Autodesk Inventor part; units mm, degrees
ref_plane "YZ Plane" through (0, 0, 0) normal (1, 0, 0) x (0, 1, 0)
ref_plane "XZ Plane" through (0, 0, 0) normal (0, 1, 0) x (-1, 0, 0)
ref_plane "XY Plane" through (0, 0, 0) normal (0, 0, 1) x (1, 0, 0)
sketch "Sketch1" plane through (0, 0, 0) normal (0, 0, 1) x (1, 0, 0)
  line L0 (-7, 0) -> (7, 0) construction
  line L1 (0, -2.8) -> (0, 2.8) construction
  line L2 (5, -2) -> (-5, -2)
  line L3 (-5, -2) -> (-5, 2)
  line L4 (-5, 2) -> (5, 2)
  line L5 (5, 2) -> (5, -2)
  line L6 (5, -2) -> (-5, 2) construction
  line L7 (-5, -2) -> (5, 2) construction
  point P0 (0, 0)
  dimension "d8" = 4
  dimension "d9" = 10
extrude "Extrusion1" add sketch "Sketch1" along normal blind 5
sketch "Sketch2" plane through (-5, 2, 0) normal (0, 1, 0) x (1, 0, 0)
  line L0 (10, 0) -> (10, -5)
  line L1 (10, 0) -> (0, 0)
  point P0 (5, 0)
  point P1 (7.5, -2.5)
  point P2 (10, -2.5)
  dimension "d12" = 2.5
hole "Hole1" at (2.5, 2, 2.5) direction (0, -1, 0) diameter 2.5 depth 10 tip angle 118 counterbore diameter 4 counterbore depth 2
sketch "Sketch3" plane through (-5, -2, 0) normal (0, -1, 0) x (1, 0, 0)
  circle A0 centre (7.5, 2.5) radius 1.25
  point P0 (5, 0)
  point P1 (2.5, 2.5)
  dimension "d21" = 5
hole "Hole2" at (-2.5, -2, 2.5) direction (0, 1, 0) diameter 2.5 depth 10 tip angle 118 counterbore diameter 4 counterbore depth 2
sketch "Sketch4" plane through (-5, 2, 0) normal (0, 1, 0) x (1, 0, 0)
  line L0 (0, 0) -> (0, -5)
  arc A0 (-12.5, 3.2297) -> (0, -2.5) centre (0, 14) ccw construction
  arc A1 (-14.3939, 1.5978) -> (0, -5) centre (0, 14) ccw
  arc A2 (-10.6061, 4.8615) -> (0, 0) centre (0, 14) ccw
  arc A3 (-10.6061, 4.8615) -> (-14.3939, 1.5978) centre (-12.5, 3.2297) ccw construction
  line L1 (10, 0) -> (0, 0)
  line L2 (10, -5) -> (0, -5)
  arc A4 (-12.5, 3.2297) -> (-27.5, 9.5) centre (-26.2704, -8.6352) ccw construction
  arc A5 (-10.6061, 4.8615) -> (-27.6691, 11.9943) centre (-26.2704, -8.6352) ccw
  arc A6 (-14.3939, 1.5978) -> (-27.3309, 7.0057) centre (-26.2704, -8.6352) ccw
  arc A7 (-14.3939, 1.5978) -> (-10.6061, 4.8615) centre (-12.5, 3.2297) ccw construction
  arc A8 (-27.6691, 11.9943) -> (-27.3309, 7.0057) centre (-27.5, 9.5) ccw
  circle A9 centre (2.5, -2.5) radius 1.25
  circle A10 centre (-27.5, 9.5) radius 1.75
  point P0 (5, 0)
  point P1 (0, 0)
  point P2 (-14.3939, 1.5978)
  point P3 (0, -5)
  dimension "d30" = 15
  dimension "d31" = 15
  dimension "d32" = 12
  dimension "d33" = 14
  dimension "d34" = 3.5
extrude "Extrusion2" add sketch "Sketch4" against normal blind 4 contours L0 A1 A6 A8 A5 A2
properties part number "huzo1"
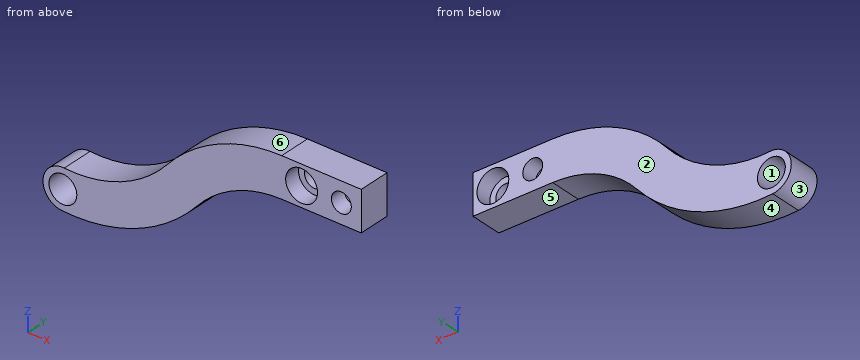
The model under review builds one solid part; all positions refer to its coordinate system, in mm. Face numbers are marked on the shaded views. A direction names the side the tool comes from. Coordinates: 2 decimals unless noted, no trailing zeros. Order: outer loops, then holes, each group sorted by start corner. A loop starts at its lowest first (then second) coordinate and runs counter-clockwise, first axis right, second up. Notation, with made-up numbers: (33.25, 7.5) -> (84.25, 7.5) arc R10 cw to (84.25, 14.5) -> close; hole circle Ø4 at (-12.5, 62). An arc over 180 degrees is marked (long way). Answer in a Markdown table with one row per item. Add a question column.
Item 1: We need section D-D on z = -8.5. Write out the cut boundary in (x, y).
Item 2: Machinability: for the marked faces 5 and 6, which of the approach directions +Z, -Z, +X, -X, +Y, -Y give a long, thin tool a straight path to every point of the face, cutting with its end or side? Answer none if there is none.
Item 3: We need section B-B on z = 2.5. Write out the cut boundary in (x, y), plus the area to 3 significant figures.
Item 4: Clearance check with flat-ended pins moving along their axes: pin 1 (1.5 mm diameter, centred on x = -17, z = 1.5, fed in from +Y); pin 2 (1.2 mm diameter, centred on x = 2.5, z = 1.5, fed in from +Y); pin 3 (3.5 mm diameter, centred on x = -2.5, z = 2.5, fed in from -Y); pin 4 (1.5 mm diameter, centred on y = 0.5, z = -7, fed in from -X). State where each tip first meets the part, or that it passes through.
Item 5: To check wall thickness, follow probe 1 along X at (y, z) = (1.2, 2.5); probe 2 along X at (y, z) = (0.5, 2); probe 3 along Z at (x, y) = (-32.5, 0.85). State the ranges of each line that lie inside material, in increasing order.
Item 6: Mouldability with a two-part tool opening along Z and no side actions: class the marked faces 1, 2, 3 and 4 as +Z half, -Z half, draft (parallel to the pull), parting line (faces both ways), or undercut.
Item 7: We need section A-A on x = 2.5. Write out the cut boundary in (y, z), plus the area to 3 significant figures.
Item 8: We need section C-C on y = 1.45. Write out the cut boundary in (x, z), plus the area to 3 significant figures.
Final values:
| question | item | result |
|---|---|---|
| 1 | outline | (-34.79, -2) -> (-33.94, -2) -> (-33.94, 2) -> (-34.79, 2) -> close; (-31.06, -2) -> (-19.7, -2) -> (-19.7, 2) -> (-31.06, 2) -> close |
| 2 | face 5 | -Z, +X, +Y, -Y |
| 2 | face 6 | +Z, -X, +Y, -Y |
| 3 | outline | (-14.42, -2) -> (-4.5, -2) -> (-4.5, 0) -> (-3.75, 0) -> (-3.75, 2) -> (-14.42, 2) -> close; (-1.25, 0) -> (-0.5, 0) -> (-0.5, -2) -> (1.25, -2) -> (1.25, 0) -> (0.5, 0) -> (0.5, 2) -> (-1.25, 2) -> close; (3.75, -2) -> (5, -2) -> (5, 2) -> (4.5, 2) -> (4.5, 0) -> (3.75, 0) -> close |
| 3 | area | 51.7 mm2 |
| 4 | pin 1 | stops at y = 2 |
| 4 | pin 2 | stops at y = 0 |
| 4 | pin 3 | stops at y = 0 |
| 4 | pin 4 | stops at x = -34.29 |
| 5 | probe 1 | x = -14.42 to -3.75, -1.25 to 0.5, 4.5 to 5 |
| 5 | probe 2 | x = -15.25 to -3.65, -1.35 to 0.56, 4.44 to 5 |
| 5 | probe 3 | z = -12.01 to -11.25, -7.75 to -7 |
| 6 | face 1 | undercut |
| 6 | face 2 | draft |
| 6 | face 3 | parting line |
| 6 | face 4 | -Z half |
| 7 | outline | (-2, 0) -> (2, 0) -> (2, 0.5) -> (0, 0.5) -> (0, 1.25) -> (-2, 1.25) -> close; (-2, 3.75) -> (0, 3.75) -> (0, 4.5) -> (2, 4.5) -> (2, 5) -> (-2, 5) -> close |
| 7 | area | 7.00 mm2 |
| 8 | outline | (-32.67, -11.99) arc R20.68 ccw to (-15.61, -4.86) arc R14 cw to (-5, 0) -> (5, 0) -> (5, 5) -> (-5, 5) arc R19 ccw to (-19.39, -1.6) arc R15.68 cw to (-32.33, -7.01) arc R2.5 ccw to start; hole circle Ø3.5 at (-32.5, -9.5); hole circle Ø2.5 at (-2.5, 2.5); hole circle Ø4 at (2.5, 2.5) |
| 8 | area | 188 mm2 |
